```python
from build123d import *

# Parameters (mm, degrees)
F0_W     = 76.2
F0_H     = 76.2
F1_DEPTH = 6.35
F2_R     = 12.7
F3_DEPTH = 25.4
F4_R     = 6.35
F5_DEPTH = 38.1


with BuildPart() as f1:
    # F0 (on Front) → F1 (new body)
    with BuildSketch(Plane.XZ):
        with Locations((38.1, 38.1)):
            Rectangle(F0_W, F0_H)
    extrude(amount=F1_DEPTH)

    # F2 (on face) → F3 (cut)
    with BuildSketch(Plane.XZ.offset(6.35)):
        with Locations((38.1, 38.1)):
            Circle(F2_R)
    extrude(amount=-F3_DEPTH, mode=Mode.SUBTRACT)

    # F4 (on face) → F5 (join)
    with BuildSketch(Plane.XZ.offset(6.35)):
        with Locations((38.1, 17.78)):
            Circle(F4_R)
    extrude(amount=F5_DEPTH)


solid = f1.part
```
Geometry: final body of the model. Coordinates: model frame, mm. Round coordinates to 2 decimals unless told otherwise and drop trailing zeros. Loops run counter-clockwise (first coordinate to the right, second up) from the corner with the lowest first, then second, coordinate; pieces in that order, holes last. Notation, with made-up numbers: (32.25, 22.5) -> (82.25, 22.5) arc R27 ccw to (82.25, 55.5) -> close; hole circle Ø2 at (-17.5, 15.5). An arc over 180 degrees is marked (long way). Write each question's results on one line, items separated by ' | '.
Item 1: Pin query (flat end, axial travel): pin 1 Ø2 at (x, y) = (44, -30) entering from -Z; pin 2 Ø1 at (x, y) = (40.5, -7.5) entering from +Z; pin 3 Ø10 at (x, y) = (36, -28) entering from -Z; pin 4 Ø12 at (x, y) = (23.5, -33) entering from +Z. Return the tip coordinate at first contact, or that it passes through.
Answers below:
pin 1: stops at z = 13.74 | pin 2: stops at z = 23.84 | pin 3: stops at z = 11.43 | pin 4: passes through
Item 2: Line query: probe 1 along X at (y, z) = (-2, 38); probe 2 along Y at (x, z) = (36.5, 52.5). Output: solid intervals per line, ascending. Write a range as [from, to].
Answers below:
probe 1: x = [0, 25.4], [50.8, 76.2] | probe 2: y = [-6.35, 0]
Item 3: Pull-direction query (X, two-part tool) for faces 1 (the face through (44.927, -3.219, 48.809)), 2 (the face through (38, -6.35, 56)), 3 (the face through (33.42, -25.13, 22.07)); classes: pulls with the +X half, pulls with the -X half, needs draft (parallel to the pull), parting line crosses it, or undercut.
Answers below:
face 1: undercut | face 2: needs draft | face 3: parting line crosses it
Item 4: Cut plane D-D on z = 17.78. Return the cut outline in (x, y), and give its area (3 significant figures).
Answers below:
outline: (0, -6.35) -> (31.75, -6.35) -> (31.75, -44.45) -> (44.45, -44.45) -> (44.45, -6.35) -> (76.2, -6.35) -> (76.2, 0) -> (0, 0) -> close | area: 968 mm²
Item 5: Cut plane A-A on x = 38.1. Return the cut outline in (y, z).
Answers below:
outline: (-44.45, 11.43) -> (-6.35, 11.43) -> (-6.35, 0) -> (0, 0) -> (0, 25.4) -> (-6.35, 25.4) -> (-6.35, 24.13) -> (-44.45, 24.13) -> close; (-6.35, 50.8) -> (0, 50.8) -> (0, 76.2) -> (-6.35, 76.2) -> close
Item 6: Cut plane C-C on y = -4. Return the cut outline in (x, z), and give its area (3 significant figures).
Answers below:
outline: (0, 0) -> (76.2, 0) -> (76.2, 76.2) -> (0, 76.2) -> close; hole circle Ø25.4 at (38.1, 38.1) | area: 5,300 mm²
Item 7: Cut plane B-B on z = 38.1. Return the cut outline in (x, y), and give its area (3 significant figures).
Answers below:
outline: (0, -6.35) -> (25.4, -6.35) -> (25.4, 0) -> (0, 0) -> close; (50.8, -6.35) -> (76.2, -6.35) -> (76.2, 0) -> (50.8, 0) -> close | area: 323 mm²
